```python
from build123d import *
from build123d.topology import SkipClean

# Parameters (mm, degrees)
SKETCH5_R            = 11.5
BOSS_EXTRUDE13_DEPTH = 598
SKETCH1_R            = 8
CUT_EXTRUDE2_DEPTH   = 17
CUT_EXTRUDE3_START   = -25
SKETCH9_R            = 8
CUT_EXTRUDE3_DEPTH   = 25
SKETCH22_R           = 29.020137942
SKETCH22_R_2         = 19
CUT_EXTRUDE4_DEPTH   = 10
SKETCH23_R           = 8
BOSS_EXTRUDE1_DEPTH  = 17
SKETCH24_R           = 11.5
BOSS_EXTRUDE2_DEPTH  = 300
SKETCH25_R           = 8
CUT_EXTRUDE5_DEPTH   = 25
BOSS_EXTRUDE3_DEPTH  = 14.86
CUT_EXTRUDE7_START   = 36
SKETCH29_R           = 21.777311072
SKETCH29_R_2         = 11.5
CUT_EXTRUDE7_DEPTH   = 36
SKETCH30_R           = 19
SKETCH30_R_2         = 11.5
CUT_EXTRUDE8_DEPTH   = 18
SKETCH27_R           = 19
BOSS_EXTRUDE9_DEPTH  = 10.03
CUT_EXTRUDE9_DEPTH   = 10.03
SKETCH35_W           = 23.953949438
SKETCH35_H           = 2.96512498
BOSS_EXTRUDE10_DEPTH = 147.5
SKETCH36_W           = 6.58
SKETCH36_H           = 5.13043091
CUT_EXTRUDE10_DEPTH  = 147.5
BOSS_EXTRUDE11_START = 5
SKETCH37_R           = 19
BOSS_EXTRUDE11_DEPTH = 5
SKETCH38_W           = 23.953949438
SKETCH38_H           = 2.96512498
CUT_EXTRUDE11_DEPTH  = 182
SKETCH39_R           = 19
SKETCH39_R_2         = 11.5
CUT_EXTRUDE12_DEPTH  = 34


with BuildPart() as part:
    # Sketch5 → Boss-Extrude13 (new body)
    with BuildSketch(Plane.XY):
        Circle(SKETCH5_R)
    extrude(amount=BOSS_EXTRUDE13_DEPTH)

    # Swept-Cut1: sweep along a path in Sketch7
    with BuildLine(Plane(origin=(0, 0, 0), x_dir=(1, 0, 0), z_dir=(0, 1, 0))) as swept_cut1_path:
        Line((11.5, -47.002601747), (-17.141789086, -39.043378107))
    # Sketch6 → Swept-Cut1 (sweep, cut)
    with BuildSketch(Plane(origin=(11.5, 0, 0), x_dir=(0, 0, -1), z_dir=(1, 0, 0))):
        Polygon((-78.362133946, 7), (-80, 11.5), (-81.283711713, 11.5), (-82.921577767, 7), (-84.645319246, 7), (-86.2831853, 11.5), (-87.566897013, 11.5), (-89.204763067, 7), (-90.928504546, 7), (-92.5663706, 11.5), (-93.850082313, 11.5), (-95.487948367, 7), (-97.211689846, 7), (-98.8495559, 11.5), (-100.133267613, 11.5), (-101.771133667, 7), (-103.494875146, 7), (-105.1327412, 11.5), (-106.416452913, 11.5), (-108.054318967, 7), (-109.778060446, 7), (-111.4159265, 11.5), (-112.699638213, 11.5), (-114.337504267, 7), (-116.061245746, 7), (-117.6991118, 11.5), (-118.982823513, 11.5), (-120.620689567, 7), (-122.344431046, 7), (-123.9822971, 11.5), (-125.266008813, 11.5), (-126.903874867, 7), (-128.627616346, 7), (-130.2654824, 11.5), (-131.549194113, 11.5), (-133.187060167, 7), (-134.910801646, 7), (-136.5486677, 11.5), (-137.832379413, 11.5), (-139.470245467, 7), (-141.193986946, 7), (-142.831853, 11.5), (-144.115564713, 11.5), (-145.753430767, 7), (-147.477172246, 7), (-149.1150383, 11.5), (-150.398750013, 11.5), (-152.036616067, 7), (-153.760357546, 7), (-155.3982236, 11.5), (-156.681935313, 11.5), (-158.319801367, 7), (-160.043542846, 7), (-161.6814089, 11.5), (-162.965120613, 11.5), (-164.602986667, 7), (-166.326728146, 7), (-167.9645942, 11.5), (-169.248305913, 11.5), (-170.886171967, 7), (-172.609913446, 7), (-174.2477795, 11.5), (-175.531491213, 11.5), (-177.169357267, 7), (-178.893098746, 7), (-180.5309648, 11.5), (-181.814676513, 11.5), (-183.452542567, 7), (-185.176284046, 7), (-186.8141501, 11.5), (-188.097861813, 11.5), (-189.735727867, 7), (-191.459469346, 7), (-193.0973354, 11.5), (-194.381047113, 11.5), (-196.018913167, 7), (-197.742654646, 7), (-199.3805207, 11.5), (-200.664232413, 11.5), (-202.302098467, 7), (-204.022098467, 7), (-206.232393599, 13.072735964), (-74.431838814, 13.072735964), (-76.642133946, 7), align=None)
    sweep(path=swept_cut1_path.line, mode=Mode.SUBTRACT)

    # Sketch11 → Revolve1 (revolve)
    with BuildSketch(Plane(origin=(0, 0, 0), x_dir=(0, 0, -1), z_dir=(1, 0, 0)), mode=Mode.PRIVATE) as revolve1_sk:
        Polygon((-380, 19), (-380, 11.5), (-390, 11.5), (-390, 14.64168316), (-387.653886088, 15.505251056), (-388.273828958, 17.92716576), (-388.161331121, 22.925900024), (-382.5, 19), align=None)
    revolve(revolve1_sk.sketch.rotate(Axis((0, 0, 0), (0, 0, 1)), 90), axis=Axis((0, 0, 0), (0, 0, 1)))

    # Sketch1 → Cut-Extrude2 (cut)
    with BuildSketch(Plane.XY.offset(598)):
        Circle(SKETCH1_R)
    extrude(amount=-CUT_EXTRUDE2_DEPTH, mode=Mode.SUBTRACT)

    # Sketch9 → Cut-Extrude3 (cut)
    with BuildSketch(Plane(origin=(0, 0, 0), x_dir=(-1, 0, 0), z_dir=(0, 0, -1)).offset(CUT_EXTRUDE3_START)):
        with Locations(Location((0, 0, 0), (0, 0, 180))):
            Circle(SKETCH9_R)
    extrude(amount=CUT_EXTRUDE3_DEPTH, mode=Mode.SUBTRACT)

    # Cut-Sweep1: sweep along a path in izim7_3
    with BuildLine(Plane(origin=(0, 0, 0), x_dir=(1, 0, 0), z_dir=(0, 1, 0))) as cut_sweep1_path:
        Line((25.154101774, -50.796919528), (-17.141789086, -39.043378107))
    # Sketch14 → Cut-Sweep1 (sweep, cut)
    with BuildSketch(Plane(origin=(11.5, 0, 0), x_dir=(0, 0, -1), z_dir=(1, 0, 0))):
        Polygon((-208.577830576, 7), (-206.368790882, 13.069286677), (-256.48542589, 13.069286677), (-306.741648428, 13.069286677), (-304.532608735, 7), (-302.812608735, 7), (-301.174742681, 11.5), (-299.891030968, 11.5), (-298.253164913, 7), (-296.529423435, 7), (-294.891557381, 11.5), (-293.607845668, 11.5), (-291.969979613, 7), (-290.246238135, 7), (-288.608372081, 11.5), (-287.324660368, 11.5), (-285.686794313, 7), (-283.963052835, 7), (-282.325186781, 11.5), (-281.041475068, 11.5), (-279.403609013, 7), (-277.679867535, 7), (-276.042001481, 11.5), (-274.758289768, 11.5), (-273.120423713, 7), (-271.396682235, 7), (-269.758816181, 11.5), (-268.475104468, 11.5), (-266.837238413, 7), (-265.113496935, 7), (-263.475630881, 11.5), (-262.191919168, 11.5), (-260.554053113, 7), (-258.830311635, 7), (-257.195219655, 11.5), (-255.915219655, 11.5), (-254.280127676, 7), (-252.556386197, 7), (-250.918520143, 11.5), (-249.63480843, 11.5), (-247.996942376, 7), (-246.273200897, 7), (-244.635334843, 11.5), (-243.35162313, 11.5), (-241.713757076, 7), (-239.990015597, 7), (-238.352149543, 11.5), (-237.06843783, 11.5), (-235.430571776, 7), (-233.706830297, 7), (-232.068964243, 11.5), (-230.78525253, 11.5), (-229.147386476, 7), (-227.423644997, 7), (-225.785778943, 11.5), (-224.50206723, 11.5), (-222.864201176, 7), (-221.140459697, 7), (-219.502593643, 11.5), (-218.21888193, 11.5), (-216.581015876, 7), (-214.857274397, 7), (-213.219408343, 11.5), (-211.93569663, 11.5), (-210.297830576, 7), align=None)
    sweep(path=cut_sweep1_path.line, mode=Mode.SUBTRACT)

    # Sketch22 → Cut-Extrude4 (cut)
    with BuildSketch(Plane(origin=(0, 0, 380), x_dir=(-1, 0, 0), z_dir=(0, 0, -1))):
        Circle(SKETCH22_R)
        Circle(SKETCH22_R_2, mode=Mode.SUBTRACT)
    extrude(amount=-CUT_EXTRUDE4_DEPTH, mode=Mode.SUBTRACT)

    # Sketch23 → Boss-Extrude1 (add)
    with BuildSketch(Plane.XY.offset(598)):
        with Locations(Location((0, 0, 0), (0, 0, 180))):
            Circle(SKETCH23_R)
    extrude(amount=-BOSS_EXTRUDE1_DEPTH)

    # Sketch24 → Boss-Extrude2 (add)
    with BuildSketch(Plane.XY.offset(598)):
        with Locations(Location((0, 0, 0), (0, 0, 180))):
            Circle(SKETCH24_R)
    extrude(amount=BOSS_EXTRUDE2_DEPTH)

    # Sketch25 → Cut-Extrude5 (cut)
    with BuildSketch(Plane.XY.offset(898)):
        with Locations(Location((0, 0, 0), (0, 0, 180))):
            Circle(SKETCH25_R)
    extrude(amount=-CUT_EXTRUDE5_DEPTH, mode=Mode.SUBTRACT)

    # Sketch26 → Boss-Extrude3 (add)
    with BuildSketch(Plane(origin=(0, 0, 380), x_dir=(-1, 0, 0), z_dir=(0, 0, -1))):
        with BuildLine():
            ThreePointArc((0.243811626, 18.825934841), (-13.39898566, -13.226581192), (18.827513557, 0))
            ThreePointArc((18.827513557, 0), (13.39898566, 13.226581192), (0.243811626, 18.825934841))
        make_face()
        with BuildLine():
            ThreePointArc((15.805163127, 7.71617291), (-10.992581615, -14.686603394), (1.492833529, 17.934216921))
            Line((1.492833529, 17.934216921), (15.805163127, 7.71617291))
        make_face(mode=Mode.SUBTRACT)
    extrude(amount=BOSS_EXTRUDE3_DEPTH)

    # Sketch29 → Cut-Extrude7 (cut)
    with BuildSketch(Plane(origin=(0, 0, 380), x_dir=(-1, 0, 0), z_dir=(0, 0, -1)).offset(CUT_EXTRUDE7_START)):
        Circle(SKETCH29_R)
        Circle(SKETCH29_R_2, mode=Mode.SUBTRACT)
    extrude(amount=-CUT_EXTRUDE7_DEPTH, mode=Mode.SUBTRACT)

    # Sketch30 → Cut-Extrude8 (cut)
    with SkipClean():  # the faces are left unmerged after this step: merging them gives an invalid solid
        with BuildSketch(Plane(origin=(0, 0, 380), x_dir=(-1, 0, 0), z_dir=(0, 0, -1))):
            Circle(SKETCH30_R)
            with Locations(Location((0, 0, 0), (0, 0, 180))):
                Circle(SKETCH30_R_2, mode=Mode.SUBTRACT)
        extrude(amount=-CUT_EXTRUDE8_DEPTH, mode=Mode.SUBTRACT)
    add(part.part.scale(1), mode=Mode.REPLACE)  # the faces are merged on a copy

    # Sketch27 → Boss-Extrude9 (add)
    with BuildSketch(Plane(origin=(0, 0, 631.57), x_dir=(-1, 0, 0), z_dir=(0, 0, -1))):
        Circle(SKETCH27_R)
    extrude(amount=-BOSS_EXTRUDE9_DEPTH)

    # Sketch33 → Cut-Extrude9 (cut)
    with BuildSketch(Plane.XY.offset(641.6)):
        with BuildLine():
            Line((-11.294482638, 15.278568714), (12.937932633, 15.278568714))
            ThreePointArc((12.937932633, 15.278568714), (0.821724997, 27.394776349), (-11.294482638, 15.278568714))
        make_face()
    extrude(amount=-CUT_EXTRUDE9_DEPTH, mode=Mode.SUBTRACT)

    # Sketch35 → Boss-Extrude10 (add)
    with BuildSketch(Plane.XY.offset(641.6)):
        with Locations((0.682492081, 16.761131204)):
            Rectangle(SKETCH35_W, SKETCH35_H)
    extrude(amount=-BOSS_EXTRUDE10_DEPTH)

    # Sketch36 → Cut-Extrude10 (cut)
    with BuildSketch(Plane(origin=(12.6594668, 0, 0), x_dir=(0, 0, -1), z_dir=(1, 0, 0))):
        with Locations((-497.39, 17.843784169)):
            Rectangle(SKETCH36_W, SKETCH36_H)
    extrude(amount=-CUT_EXTRUDE10_DEPTH, mode=Mode.SUBTRACT)

    # Sketch37 → Boss-Extrude11 (add)
    with BuildSketch(Plane(origin=(0, 0, 500.68), x_dir=(-1, 0, 0), z_dir=(0, 0, -1)).offset(BOSS_EXTRUDE11_START)):
        with Locations(Location((0, 0, 0), (0, 0, 126.47318116))):
            Circle(SKETCH37_R)
    extrude(amount=-BOSS_EXTRUDE11_DEPTH)

    # Sketch38 → Cut-Extrude11 (cut)
    with BuildSketch(Plane(origin=(0, 0, 500.68), x_dir=(-1, 0, 0), z_dir=(0, 0, -1))):
        with Locations((-0.682492081, 16.761131204)):
            Rectangle(SKETCH38_W, SKETCH38_H)
    extrude(amount=-CUT_EXTRUDE11_DEPTH, mode=Mode.SUBTRACT)

    # Sketch39 → Cut-Extrude12 (cut)
    with BuildSketch(Plane(origin=(0, 0, 631.57), x_dir=(-1, 0, 0), z_dir=(0, 0, -1))):
        Circle(SKETCH39_R)
        Circle(SKETCH39_R_2, mode=Mode.SUBTRACT)
    extrude(amount=-CUT_EXTRUDE12_DEPTH, mode=Mode.SUBTRACT)


solid = part.part
```
The model under review builds one solid part; all positions refer to its coordinate system, in mm. A direction names the side the tool comes from. Round coordinates to 2 decimals unless told otherwise and drop trailing zeros. Loops run counter-clockwise (first coordinate to the right, second up) from the corner with the lowest first, then second, coordinate; pieces in that order, holes last.
1) Clearance check with flat-ended pins moving along their axes: P1, Ø5, axis at x = -3.5, z = 477, coming from the +Y side; P2, Ø3.5, axis at x = -4.5, z = 138.5, coming from the +Y side; P3, Ø8, axis at x = 1.5, y = 3, coming from the +Z side. State where each tip first meets the part, or that it passes through.
Values follow:
P1: stops at y = 11.46
P2: stops at y = 11.16
P3: stops at z = 873
2) Tool access review of faces 4 (the face through (0, 0, 873)), 5 (the face through (-2, -8, 898)), 6 (the face through (-1.73, 7.81, 12.68)): name each direction out of +Z, -Z, +X, -X, +Y, -Y from which nothing blocks a thin tool from reaching the whole face with its end or side.
Values follow:
face 4: +Z
face 5: +Z, +X, -X, +Y, -Y
face 6: -Z
3) Consider section A-A on z = 543.5. State the section outline as (x, y) points, then the cut area to 3 significant figures.
Values follow:
outline: circle Ø23 at (0, 0)
area: 415 mm2
4) Wall thickness on line 1 along Y through (x, z) = (0, 881); line 2 along Y through (x, z) = (7, 647); line 3 along Z through (x, y) = (13, 7): over which ranges is each line inside the solid? List them lowest first.
Values follow:
line 1: y = -11.5 to -8, 8 to 11.5
line 2: y = -9.12 to 9.12
line 3: z = 495.68 to 500.68
5) The part is to be moulded in two halves that separate along Y. For faces 1 (the face through (-18.26, -5.25, 498.14)), 2 (the face through (-8, -2, 0)), 3 (the face through (0, 0, 25)), say which applies: pulls with the +Y half, pulls with the -Y half, needs draft (parallel to the pull), parting line crosses it, or undercut.
Values follow:
face 1: parting line crosses it
face 2: needs draft
face 3: undercut
